Geometry check sheet. Reference: the model listing, model coordinates, mm. Round coordinates to 2 decimals unless told otherwise and drop trailing zeros. Write each loop counter-clockwise with the first axis right and the second up, starting at its lowest first coordinate (ties: lowest second). Pieces come first, ordered by that corner, then holes.
Autodesk Inventor part; units mm, degrees
ref_plane "Work Plane1" through (0, 0, 0) normal (0, 0, 1) x (1, 0, 0)
ref_plane "YZ Plane" through (0, 0, 0) normal (1, 0, 0) x (0, 1, 0)
ref_plane "XZ Plane" through (0, 0, 0) normal (0, 1, 0) x (-1, 0, 0)
sketch "Sketch1" plane through (0, 0, 0) normal (0, 0, 1) x (1, 0, 0)
  circle A0 centre (0, 0) radius 4.375
  circle A1 centre (0, 0) radius 4.4
  dimension "d1" = 8.75
  dimension "d2" = 8.8
extrude "Extrusion1" add sketch "Sketch1" along normal mid plane 2.8
ref_plane "Work Plane1" through (0, 0, 0) normal (0, 0, 1) x (1, 0, 0)
sketch "Sketch2" plane through (0, 0, 0) normal (0, 0, 1) x (1, 0, 0)
  circle A0 centre (0, 4.3875) radius 0.5
  circle A1 centre (-2.1937, 3.7997) radius 0.5
  circle A2 centre (-3.7997, 2.1938) radius 0.5
  circle A3 centre (-4.3875, 0) radius 0.5
  circle A4 centre (-3.7997, -2.1937) radius 0.5
  circle A5 centre (-2.1938, -3.7997) radius 0.5
  circle A6 centre (0, -4.3875) radius 0.5
  circle A7 centre (2.1937, -3.7997) radius 0.5
  circle A8 centre (3.7997, -2.1938) radius 0.5
  circle A9 centre (4.3875, 0) radius 0.5
  circle A10 centre (3.7997, 2.1938) radius 0.5
  circle A11 centre (2.1937, 3.7997) radius 0.5
  point P0 (0, 0)
  dimension "d5" = 1
  dimension "d6" = 4.3875
  dimension "d9" = 360
extrude "Extrusion2" cut sketch "Sketch2" along normal mid plane 2
properties part number "Lock"
1. Depth check by flat-ended pin: pin 1 Ø1.5 at (x, z) = (2, -0.5) entering from -Y. Enter the tip coordinate at first touch or a pass-through.
2. Section check D-D (z = 0.65). State how many separate pieces and enclosed holes the cut face has, plus the area to 3 significant figures.
3. Section check A-A (y = 0). Record the cut outline in (x, z) (3 decimals).
Results below:
1. pin 1: stops at y = -4.22
2. separate pieces: 12
2. enclosed holes: 0
2. area: 0.389 mm2
3. outline: (-4.4, -1.4) - (-4.375, -1.4) - (-4.375, -1) - (-4.4, -1) - close; (-4.4, 1) - (-4.375, 1) - (-4.375, 1.4) - (-4.4, 1.4) - close; (4.375, -1.4) - (4.4, -1.4) - (4.4, -1) - (4.375, -1) - close; (4.375, 1) - (4.4, 1) - (4.4, 1.4) - (4.375, 1.4) - close
